Here's the drawing with two shaded views (mm, measured from the low corner). I have some questions. Coordinates: 2 decimals unless noted, no trailing zeros. Write each loop counter-clockwise with the first axis right and the second up, starting at its lowest first coordinate (ties: lowest second). Pieces come first, ordered by that corner, then holes.
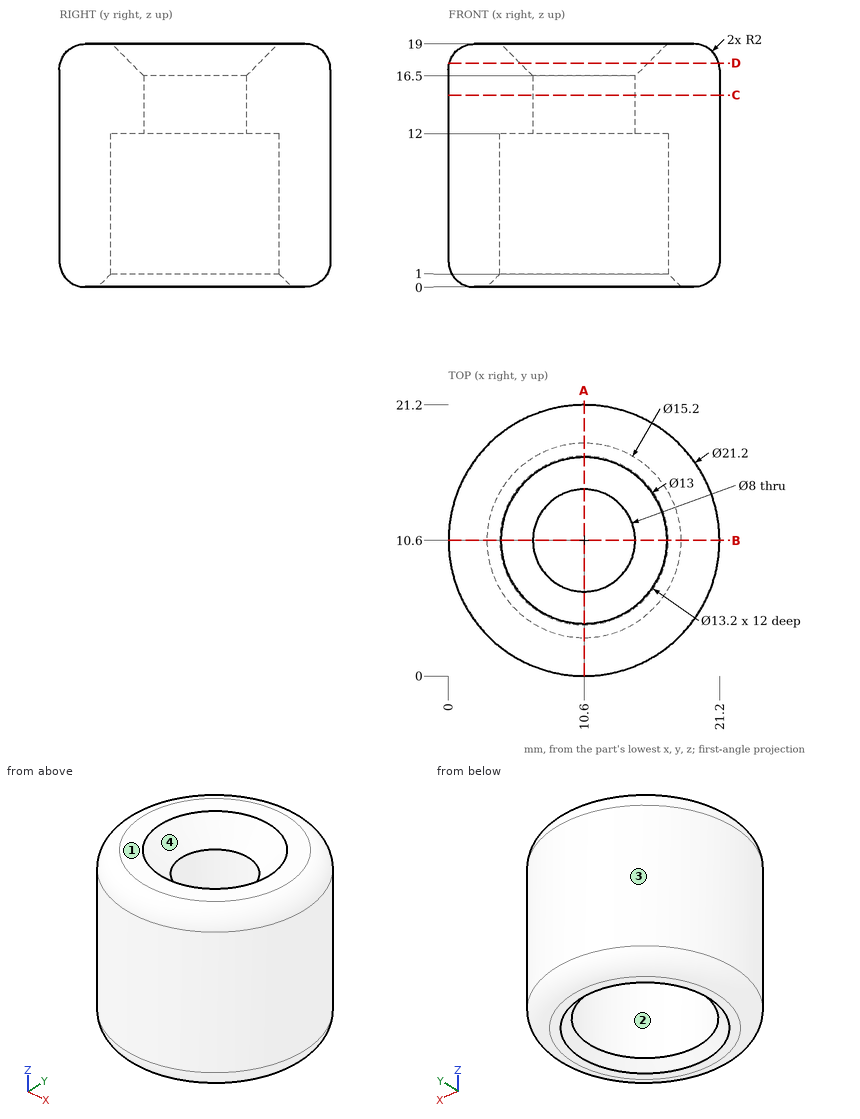
Item 1: If we mould it in two halves opening along X, with no side actions, what happens to the marked faces 1, 2, 3 and 4? For each: released by +X, released by -X, zero draft, split by the parting line, or undercut.
Item 2: Will these pins go through, and if not, where does the flat tip stop? pin 1 Ø5 at (x, y) = (10.6, 10.6) entering from -Z; pin 2 Ø1.5 at (y, z) = (4, 16.5) entering from -X; pin 3 Ø2 at (y, z) = (17, 5.5) entering from -X; pin 4 Ø1.5 at (x, y) = (14.5, 11.5) entering from +Z.
Item 3: I want a section at A-A, the plane x = 10.6. List the corners of the cut face in (y, z) for me, then the cut area to 3 significant figures.
Item 4: If I drill on line 1 along Y through (x, z) = (10.6, 13.2); line 2 along Y through (x, z) = (10.6, 7.5); line 3 along X through (y, z) = (15.75, 9.75), over which ranges is the centre line in solid material (lowest first)?
Item 5: I want a section at D-D, the plane z = 17.5. List the corners of the cut face in (x, y) for me, then the cut area to 3 significant figures.
Item 6: I want a section at C-C, the plane z = 15. List the corners of the cut face in (x, y) for me, then the cut area to 3 significant figures.
Taken from the geometry:
1. face 1: zero draft
1. face 2: undercut
1. face 3: split by the parting line
1. face 4: undercut
2. pin 1: passes through
2. pin 2: stops at x = 1.76
2. pin 3: stops at x = 1.48
2. pin 4: stops at z = 17.25
3. outline: (0, 2) arc R2 ccw to (2, 0) - (3, 0) - (4, 1) - (4, 12) - (6.6, 12) - (6.6, 16.5) - (4.1, 19) - (2, 19) arc R2 ccw to (0, 17) - close; (14.6, 12) - (17.2, 12) - (17.2, 1) - (18.2, 0) - (19.2, 0) arc R2 ccw to (21.2, 2) - (21.2, 17) arc R2 ccw to (19.2, 19) - (17.1, 19) - (14.6, 16.5) - close
3. area: 178 mm2
4. line 1: y = 0 to 6.6, 14.6 to 21.2
4. line 2: y = 0 to 4, 17.2 to 21.2
4. line 3: x = 1.34 to 6.47, 14.73 to 19.86
5. outline: circle Ø21.07 at (10.6, 10.6); hole circle Ø10 at (10.6, 10.6)
5. area: 270 mm2
6. outline: circle Ø21.2 at (10.6, 10.6); hole circle Ø8 at (10.6, 10.6)
6. area: 303 mm2
